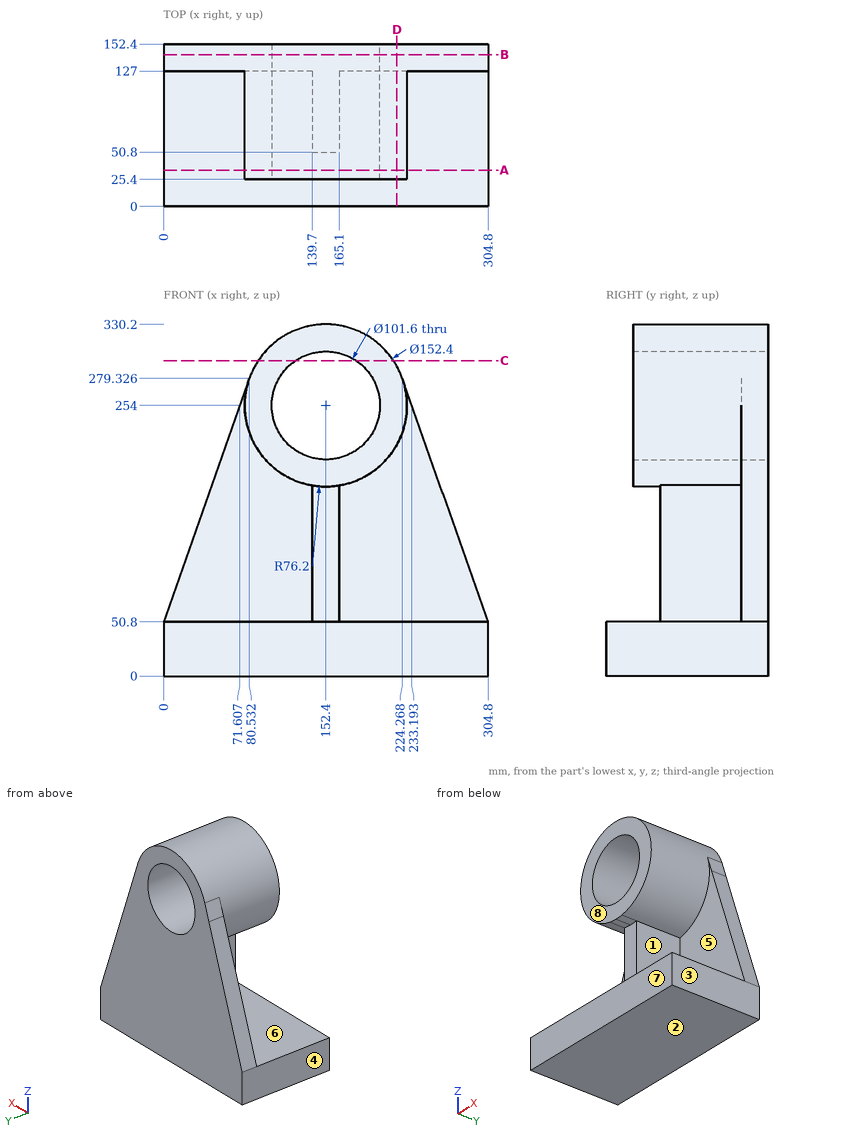
Check sheet for the drawn part. Datum: minimum x, y, z corner. Units: mm. A direction names the side the tool comes from. Give positions to 0.01 mm unless a question says otherwise; leave off trailing zeros. Write each loop counter-clockwise with the first axis right and the second up, starting at its lowest first coordinate (ties: lowest second). Pieces come first, ordered by that corner, then holes.
(1) Mould release check, pull along Z, two halves, no side actions. Record for the marked faces 1, 2 and 3: +Z half, -Z half, draft (parallel to the pull), parting line (faces both ways), or undercut.
(2) Cross-section at D-D (x = 219). Enter the section's corners in (y, z).
(3) Cross-section at C-C (z = 296). Enter the section's corners in (x, y).
(4) Cross-section at B-B (y = 142.5). Enter the section's corners in (x, z), plus the area to 3 significant figures.
(5) Gauge pin test, flat ends, axial feed: pin 1 (3 mm diameter, centred on y = 67, z = 67, fed in from +X); pin 2 (7.5 mm diameter, centred on x = 157.5, z = 117, fed in from -Y); pin 3 (10 mm diameter, centred on y = 19, z = 210, fed in from +X). Record the tip position at first contact, or that the pin passes through.
(6) Cross-section at A-A (y = 34). Enter the section's corners in (x, z).
(7) Material ranges on line 1 (Z direction, x = 152.4, y = 102); line 2 (Z direction, x = 106.5, y = 107) (1 decimal); line 3 (Y direction, x = 128, z = 122), recorded low to high.
(8) Access from +Z, -Z, +X, -X, +Y, -Y to the whole of each face (thin tool, end or side, straight path). Record for the marked faces 4, 5, 6, 7 and 8.
Worked out:
1. face 1: undercut
1. face 2: -Z half
1. face 3: draft
2. outline: (0, 0) - (152.4, 0) - (152.4, 291.03) - (25.4, 291.03) - (25.4, 216.97) - (127, 216.97) - (127, 50.8) - (0, 50.8) - close
3. outline: (88.82, 25.4) - (123.82, 25.4) - (123.82, 152.4) - (88.82, 152.4) - close; (180.98, 25.4) - (215.98, 25.4) - (215.98, 152.4) - (180.98, 152.4) - close
4. outline: (0, 0) - (304.8, 0) - (304.8, 50.8) - (224.27, 279.33) arc R76.2 ccw to (80.53, 279.33) - (0, 50.8) - close; hole circle Ø101.6 at (152.4, 254)
4. area: 64,000 mm2
5. pin 1: stops at x = 165.1
5. pin 2: stops at y = 50.8
5. pin 3: passes through
6. outline: (0, 0) - (304.8, 0) - (304.8, 50.8) - (0, 50.8) - close; circle Ø152.4 at (152.4, 254); hole circle Ø101.6 at (152.4, 254)
7. line 1: z = 0 to 203.2, 304.8 to 330.2
7. line 2: z = 0 to 50.8, 193.2 to 232.2, 275.8 to 314.8
7. line 3: y = 127 to 152.4
8. face 4: +Z, -Z, -X, +Y, -Y
8. face 5: +X, -Y
8. face 6: -Y
8. face 7: +Z, -Z, +X, -X, -Y
8. face 8: +Z, +X, -X, -Y
